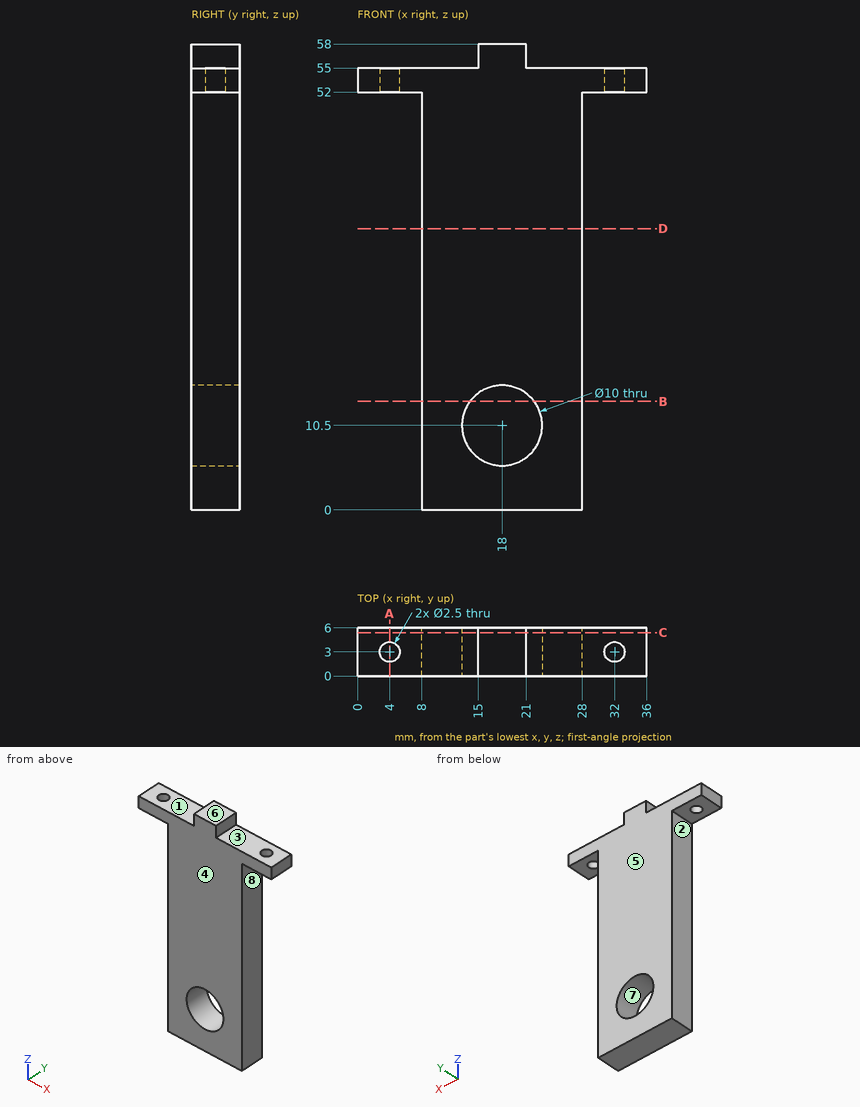
Geometry: see drawing. Coordinates: mm, zero at the bounding-box minimum. A direction names the side the tool comes from. Give positions to 0.01 mm unless a question says otherwise; leave off trailing zeros. Write each loop counter-clockwise with the first axis right and the second up, starting at its lowest first coordinate (ties: lowest second). Pieces come first, ordered by that corner, then holes. Notation, with made-up numbers: (-15, 0.5) -> (22, 0.5) arc R16 cw to (22, 23.5) -> close; hole circle Ø2 at (77, -39.75). An arc over 180 degrees is marked (long way). Use one line per item in the form item = value. Start each with the question number.
1) Ray query, probe 1 along X at (y, z) = (3, 53.55); probe 2 along X at (y, z) = (4, 10.5); probe 3 along X at (y, z) = (2.4, 54.5). Return the intervals inside material, ascending. Write a range as from..to.
2) Set-up query: the marked faces 1, 2, 3, 4 and 5. Return all of +Z, -Z, +X, -X, +Y, -Y with unobstructed straight access to the full face (end or side cutting, diameter ignored); none if empty.
3) Pin query (flat end, axial travel): pin 1 (12 mm diameter, centred on x = 7.5, z = 16.5, fed in from +Y); pin 2 (1.8 mm diameter, centred on y = 2.5, z = 28.5, fed in from -X); pin 3 (2.5 mm diameter, centred on y = 2.5, z = 56.5, fed in from -X); pin 4 (3 mm diameter, centred on x = 3.5, y = 2.5, fed in from -Z). Return the tip coordinate at first contact, or that it passes through.
4) Section query A-A on x = 4. Return the cut outline in (y, z).
5) Draft query along X for the marked faces 6, 7 and 8. Return one class per face: pulls with the +X half, pulls with the -X half, needs draft (parallel to the pull), parting line crosses it, or undercut.
6) Section query B-B on z = 13.5. Return the cut outline in (x, y), then the cut area to 3 significant figures.
7) Section query D-D on z = 35. Return the cut outline in (x, y), then the cut area to 3 significant figures.
8) Section query C-C on y = 5.4. Return the cut outline in (x, z), then the cut area to 3 significant figures.
Outcome:
q1.probe_1 = 0..2.75, 5.25..30.75, 33.25..36
q1.probe_2 = 8..13, 23..28
q1.probe_3 = 0..2.9, 5.1..30.9, 33.1..36
q2.face_1 = +Z, -X, +Y, -Y
q2.face_2 = -Z, -X, +Y, -Y
q2.face_3 = +Z, +X, +Y, -Y
q2.face_4 = +Z, -Z, +X, -X, -Y
q2.face_5 = +Z, -Z, +X, -X, +Y
q3.pin_1 = 6
q3.pin_2 = 8
q3.pin_3 = 15
q3.pin_4 = 52
q4.outline = (0, 52) -> (1.75, 52) -> (1.75, 55) -> (0, 55) -> close; (4.25, 52) -> (6, 52) -> (6, 55) -> (4.25, 55) -> close
q5.face_6 = needs draft
q5.face_7 = undercut
q5.face_8 = pulls with the +X half
q6.outline = (8, 0) -> (14, 0) -> (14, 6) -> (8, 6) -> close; (22, 0) -> (28, 0) -> (28, 6) -> (22, 6) -> close
q6.area = 72.0 mm^2
q7.outline = (8, 0) -> (28, 0) -> (28, 6) -> (8, 6) -> close
q7.area = 120 mm^2
q8.outline = (0, 52) -> (8, 52) -> (8, 0) -> (28, 0) -> (28, 52) -> (36, 52) -> (36, 55) -> (21, 55) -> (21, 58) -> (15, 58) -> (15, 55) -> (0, 55) -> close; hole circle Ø10 at (18, 10.5)
q8.area = 1,090 mm^2
